Can you work these out from the model? Positions are in its coordinate system, mm. A direction names the side the tool comes from. Give positions to 0.01 mm unless a question says otherwise; leave off trailing zeros. Write each loop counter-clockwise with the first axis right and the second up, starting at its lowest first coordinate (ties: lowest second). Pieces come first, ordered by that corner, then holes.
Autodesk Inventor part; units mm, degrees
ref_plane "YZ Plane" through (0, 0, 0) normal (1, 0, 0) x (0, 1, 0)
ref_plane "XZ Plane" through (0, 0, 0) normal (0, 1, 0) x (-1, 0, 0)
ref_plane "XY Plane" through (0, 0, 0) normal (0, 0, 1) x (1, 0, 0)
sketch "Sketch1" plane through (0, 0, 0) normal (0, 0, 1) x (1, 0, 0)
  line L0 (0, 0) -> (9.8, 0)
  line L1 (9.8, 0) -> (9.8, 13.6)
  line L2 (9.8, 13.6) -> (0, 13.6)
  line L3 (0, 13.6) -> (0, 0)
  line L4 (1.575, 13.6) -> (8.225, 13.6)
  line L5 (8.225, 13.6) -> (8.225, 98.4)
  line L6 (8.225, 98.4) -> (1.575, 98.4)
  line L7 (1.575, 98.4) -> (1.575, 13.6)
  line L8 (1.575, 56) -> (8.225, 56) construction
  line L9 (0, 112) -> (9.8, 112)
  line L10 (9.8, 112) -> (9.8, 98.4)
  line L11 (9.8, 98.4) -> (0, 98.4)
  line L12 (0, 98.4) -> (0, 112)
  line L13 (1.575, 98.4) -> (8.225, 98.4)
  circle A0 centre (4.9, 6.75) radius 2
  line L14 (4.9, 6.75) -> (4.9, 56) construction
  circle A1 centre (4.9, 105.25) radius 2
  line L15 (4.9, 105.25) -> (4.9, 56) construction
  point P0 (4.9, 13.6)
  point P1 (4.9, 98.4)
  dimension "d0" = 9.8
  dimension "d1" = 13.6
  dimension "d2" = 112
  dimension "d3" = 6.65
  dimension "d6" = 4
  dimension "d7" = 98.5
extrude "Extrusion1" add sketch "Sketch1" along normal blind 6.6 contours L3 L2 L1 L0 | L7 L6 L5 L2 | L11 L12 L9 L10 L6 | A0 | A1
extrude "Extrusion2" add sketch "Sketch1" against normal blind 3.75 contours A0 | A1
sketch "Sketch2" plane through (0, 0, 6.6) normal (0, 0, 1) x (1, 0, 0)
  line L0 (0, 0) -> (9.8, 0)
  line L1 (3.7, 0) -> (6.1, 0)
  line L2 (6.1, 0) -> (6.1, 112)
  line L3 (6.1, 112) -> (3.7, 112)
  line L4 (3.7, 112) -> (3.7, 0)
  line L5 (9.8, 112) -> (0, 112)
  point P0 (4.9, 112)
  dimension "d10" = 2.4
extrude "Extrusion3" cut sketch "Sketch2" against normal blind 2.4
chamfer "Chamfer1" distance 3.5 angle 22.5 1 edges at (3.7, 112, 5.4) measured on face at (3.7, 74.6667, 5.8)
chamfer "Chamfer2" distance 3.5 angle 22.5 1 edges at (6.1, 112, 5.4) measured on face at (6.1, 37.3333, 5.8)
chamfer "Chamfer3" distance 3.5 angle 22.5 1 edges at (4.9, 112, 4.2) measured on face at (4.5, 36.1667, 4.2)
chamfer "Chamfer4" distance 3.5 angle 22.5 1 edges at (3.7, 0, 5.4) measured on face at (3.7, 36.1667, 5)
chamfer "Chamfer5" distance 3.5 angle 22.5 1 edges at (6.1, 0, 5.4) measured on face at (6.1, 36.1667, 5.8)
chamfer "Chamfer6" distance 3.5 angle 22.5 1 edges at (4.9, 0, 4.2) measured on face at (5.3, 73.5, 4.2)
properties part number "CCA Rail"
1) If we mould it in two halves opening along Y, with no side actions, what happens to faces 1 (the face through (1.575, 57, 3)), 2 (the face through (3.426, 8.102, -1.849)), 3 (the face through (2.965, 1.726, 5.076)), 4 (the face through (8, 57, 6.6))? For each: +Y half, -Y half, draft (parallel to the pull), parting line (faces both ways), or undercut.
Values follow:
face 1: undercut
face 2: undercut
face 3: -Y half
face 4: draft
2) Please list where these lines run through material, in increasing order: L1, parallel to Y at x = 1, z = 3; L2, parallel to Z at x = 7.5, y = 89; L3, parallel to X at y = 64, z = 4.25 (3 decimals).
Values follow:
L1: y = 0 to 13.6, 98.4 to 112
L2: z = 0 to 6.6
L3: x = 1.575 to 3.7, 6.1 to 8.225
3) Suppose I cut it at D-D on y = 88. Write out the boundary of the cut face in (x, z) (3 decimals), plus the area to 3 significant figures.
Values follow:
outline: (1.575, 0) - (8.225, 0) - (8.225, 6.6) - (6.1, 6.6) - (6.1, 4.2) - (3.7, 4.2) - (3.7, 6.6) - (1.575, 6.6) - close
area: 38.1 mm2
4) Suppose I cut it at A-A on z = 5.5. Write out the boundary of the cut face in (x, y) (3 decimals), plus the area to 3 significant figures.
Values follow:
outline: (0, 0) - (2.25, 0) - (3.7, 3.5) - (3.7, 108.5) - (2.25, 112) - (0, 112) - (0, 98.4) - (1.575, 98.4) - (1.575, 13.6) - (0, 13.6) - close; (6.1, 3.5) - (7.55, 0) - (9.8, 0) - (9.8, 13.6) - (8.225, 13.6) - (8.225, 98.4) - (9.8, 98.4) - (9.8, 112) - (7.55, 112) - (6.1, 108.5) - close
area: 552 mm2
5) Suppose I cut it at C-C on x = 4.9. Write out the boundary of the cut face in (y, z), plus the area to 3 significant figures.
Values follow:
outline: (0, 0) - (4.75, 0) - (4.75, -3.75) - (8.75, -3.75) - (8.75, 0) - (103.25, 0) - (103.25, -3.75) - (107.25, -3.75) - (107.25, 0) - (112, 0) - (112, 2.75) - (108.5, 4.2) - (3.5, 4.2) - (0, 2.75) - close
area: 495 mm2
6) Suppose I cut it at B-B on y = 105.25. Write out the boundary of the cut face in (x, z), plus the area to 3 significant figures.
Values follow:
outline: (0, 0) - (2.9, 0) - (2.9, -3.75) - (6.9, -3.75) - (6.9, 0) - (9.8, 0) - (9.8, 6.6) - (6.1, 6.6) - (6.1, 4.2) - (3.7, 4.2) - (3.7, 6.6) - (0, 6.6) - close
area: 73.9 mm2
7) For pin 1 Ø1.9 at (x, y) = (5, 68) entering from +Z; pin 2 Ø5 at (x, y) = (1, 63) entering from -Z; pin 3 Ø0.8 at (x, z) = (1, 4) entering from -Y; pin 4 Ø1.9 at (y, z) = (72, 5.5) entering from -X (3 decimals), each with a flat end and sliding along its axis, tell me the tip position at first contact or that it passes through.
Values follow:
pin 1: stops at z = 4.2
pin 2: stops at z = 0
pin 3: stops at y = 0
pin 4: stops at x = 1.575
8) For faces 5 (the face through (4.64, 107.233, -1.849)), 6 (the face through (8.225, 55, 3)), 7 (the face through (5, 57, 4.2)), 8 (the face through (6.835, 110.274, 5.13)), which set-ups out of +Z, -Z, +X, -X, +Y, -Y let a thin tool reach every point of the face, with its end or its side?
Values follow:
face 5: -Z
face 6: +Z, -Z, +X
face 7: +Z, +Y, -Y
face 8: +Z, +Y
